Can you work these out from the model? Positions are in its coordinate system, mm. Face numbers are marked on the shaded views. A direction names the side the tool comes from. Give positions to 0.01 mm unless a question says otherwise; leave off trailing zeros. Order: outer loops, then holes, each group sorted by start corner. A loop starts at its lowest first (then second) coordinate and runs counter-clockwise, first axis right, second up.
Autodesk Inventor part; units mm, degrees
ref_plane "Work Plane1" through (0, 0, -15) normal (0, 0, 1) x (1, 0, 0)
ref_plane "YZ Plane" through (0, 0, 0) normal (1, 0, 0) x (0, 1, 0)
ref_plane "XZ Plane" through (0, 0, 0) normal (0, 1, 0) x (-1, 0, 0)
sketch "Sketch1" plane through (0, 0, 0) normal (0, 0, 1) x (1, 0, 0)
  line L0 (0, 0) -> (25, 0)
  line L1 (25, 0) -> (25, 40)
  line L2 (25, 40) -> (0, 40)
  line L3 (0, 40) -> (0, 0)
  dimension "d1" = 25
  dimension "d2" = 40
  dimension "d3" = 25
extrude "Extrusion1" add sketch "Sketch1" against normal blind 30
sketch "Sketch2" plane through (25, 0, 0) normal (1, 0, 0) x (0, 0, -1)
  line L0 (0, 0) -> (30, 0)
  circle A0 centre (15, 6.56) radius 2.46
extrude "Extrusion2" cut sketch "Sketch2" against normal blind 30
sketch "Sketch3" plane through (0, 0, 0) normal (-1, 0, 0) x (0, 0, 1)
  line L0 (0, 0) -> (-30, 0)
  line L1 (-25.05, 0) -> (-4.95, 0)
  line L2 (-4.95, 0) -> (-4.95, 33.12)
  line L3 (-4.95, 33.12) -> (-25.05, 33.12)
  line L4 (-25.05, 33.12) -> (-25.05, 0)
  dimension "d11" = 20.1
extrude "Extrusion3" cut sketch "Sketch3" against normal blind 20
sketch "Sketch4" plane through (0, 0, 0) normal (0, -1, 0) x (1, 0, 0)
  line L0 (20, -4.95) -> (20, -25.05)
  line L1 (20, -15) -> (25, -15)
  line L2 (25, 0) -> (25, -30)
  line L3 (20, -8.025) -> (25, -8.025)
  line L4 (25, -8.025) -> (25, -21.975)
  line L5 (25, -21.975) -> (20, -21.975)
  line L6 (20, -21.975) -> (20, -8.025)
  line L7 (20, -8.025) -> (25, -21.975) construction
  line L8 (25, -8.025) -> (20, -21.975) construction
  line L9 (25, -12.54) -> (25, -17.46)
  point P0 (0, 0)
  point P1 (22.5, -15)
  dimension "d14" = 13.95
extrude "Extrusion4" add sketch "Sketch4" along normal blind 15
sketch "Sketch5" plane through (20, 0, 0) normal (-1, 0, 0) x (0, 0, 1)
  circle A0 centre (-15, 6.56) radius 2.46
  circle A1 centre (-15, 6.56) radius 4.7025
  circle A2 centre (-15, 6.56) radius 2.46
  circle A3 centre (-15, 6.56) radius 2.46
  point P0 (0, 0)
  dimension "d17" = 9.405
extrude "Extrusion5" cut sketch "Sketch5" against normal blind 2.1
sketch "Sketch6" plane through (25, 0, 0) normal (1, 0, 0) x (0, 0, -1)
  circle A0 centre (15, 6.56) radius 4.7025
  line L0 (15, 6.56) -> (15, 23.56)
  circle A1 centre (15, 23.56) radius 2.46
  point P0 (0, 0)
  dimension "d20" = 17
  dimension "d21" = 4.92
extrude "Extrusion6" cut sketch "Sketch6" against normal blind 10 contours A1
sketch "Sketch7" plane through (20, 0, 0) normal (-1, 0, 0) x (0, 0, 1)
  circle A0 centre (-15, 23.56) radius 2.46
  circle A1 centre (-15, 23.56) radius 4.7025
  point P0 (0, 0)
  dimension "d24" = 9.405
extrude "Extrusion7" cut sketch "Sketch7" against normal blind 2.1
sketch "Sketch9" plane through (25, 0, 0) normal (1, 0, 0) x (0, 0, -1)
  circle A0 centre (15, 6.56) radius 2.46
  circle A1 centre (15, 6.56) radius 2.46
  circle A2 centre (15, 23.56) radius 2.46
  circle A3 centre (15, 23.56) radius 2.46
  line L0 (30, 40) -> (30, 0)
  line L1 (30, 0) -> (30, 40)
  line L2 (30, 40) -> (0, 40)
  line L3 (0, 40) -> (0, 0)
  line L4 (0, 0) -> (8.025, 0)
  line L5 (21.975, 0) -> (21.975, -15)
  line L6 (21.975, -15) -> (8.025, -15)
  line L7 (8.025, -15) -> (8.025, 0)
  line L8 (0, 0) -> (8.025, 0)
  line L9 (21.975, 0) -> (30, 0)
extrude "Extrusion8" add sketch "Sketch9" along normal blind 5
sketch "Sketch10" plane through (0, 40, 0) normal (0, 1, 0) x (1, 0, 0)
  line L0 (0, 30) -> (30, 30)
  line L1 (30, 0) -> (0, 0)
  line L2 (0, 30) -> (30, 30)
  line L3 (30, 30) -> (30, 0)
  line L4 (30, 0) -> (0, 0)
  line L5 (0, 0) -> (0, 30)
extrude "Extrusion9" add sketch "Sketch10" along normal blind 30
sketch "Sketch12" plane through (30, 0, 0) normal (1, 0, 0) x (0, 0, -1)
  circle A0 centre (15, 6.56) radius 2.46
  line L0 (15, 6.56) -> (15, 15.06)
  circle A1 centre (15, 15.06) radius 2.525
  point P0 (0, 0)
  dimension "d31" = 8.5
  dimension "d33" = 5.05
extrude "Extrusion10" cut sketch "Sketch12" against normal blind 30 contours A1
sketch "Sketch15" plane through (0, 0, -25.05) normal (-1, 0, 0) x (0, 0, 1)
  line L0 (0, 33.12) -> (20.1, 33.12)
  line L1 (20.1, 33.12) -> (20.1, 0)
  line L2 (0, 33.12) -> (20.1, 33.12)
  line L3 (20.1, 33.12) -> (20.1, 31.1)
  line L4 (20.1, 31.1) -> (0, 31.1)
  line L5 (0, 31.1) -> (0, 33.12)
  point P0 (25.05, 0)
  dimension "d57" = 2.02
extrude "Extrusion13" add sketch "Sketch15" against normal blind 20
sketch "Sketch17" plane through (0, 0, 0) normal (0, 0, 1) x (1, 0, 0)
  line L0 (0, 70) -> (30, 70)
  line L1 (30, 70) -> (50.0622, 90.0622)
  line L2 (30, 70) -> (80, 70) construction
  line L3 (11.9522, 97.2454) -> (0, 85.2932)
  line L4 (0, 70) -> (0, 85.2932)
  line L5 (0, 70) -> (0, 0)
  line L6 (0, 70) -> (30, 70)
  line L7 (10.923, 112.2849) -> (0, 120.567)
  line L8 (50.0622, 105.3553) -> (50.0622, 120.567)
  line L9 (50.0622, 105.3553) -> (50.0622, 90.0622)
  arc A0 (11.9522, 97.2454) -> (10.923, 112.2849) centre (4.8811, 104.3165) ccw
  line L10 (0, 165.567) -> (30, 165.567)
  line L11 (30, 165.567) -> (50.0622, 120.567)
  line L12 (6, 163.067) -> (0, 165.567)
  line L13 (6, 123.067) -> (0, 120.567)
  line L14 (6, 123.067) -> (12, 143.067)
  line L15 (12, 143.067) -> (6, 163.067)
  dimension "d61" = 45
  dimension "d62" = 32.0271
  dimension "d72" = 10
extrude "Extrusion14" add sketch "Sketch17" against normal blind 30
sketch "Sketch24" plane through (0, 0, 0) normal (0, 0, 1) x (1, 0, 0)
  line L0 (30, 70) -> (50.0622, 90.0622)
  line L1 (30, 70) -> (50.0622, 90.0622)
  line L2 (50.0622, 90.0622) -> (50.0622, 120.567)
  line L3 (50.0622, 90.0622) -> (50.0622, 120.567)
  line L4 (30, 165.567) -> (50.0622, 120.567)
  line L5 (50.0622, 120.567) -> (30, 165.567)
  line L6 (0, 165.567) -> (30, 165.567)
  line L7 (30, 165.567) -> (0, 165.567)
  line L8 (6, 163.067) -> (0, 165.567)
  line L9 (0, 165.567) -> (6, 163.067)
  line L10 (12, 143.067) -> (6, 163.067)
  line L11 (6, 163.067) -> (12, 143.067)
  line L12 (6, 123.067) -> (12, 143.067)
  line L13 (12, 143.067) -> (6, 123.067)
  line L14 (0, 120.567) -> (6, 123.067)
  line L15 (6, 123.067) -> (0, 120.567)
  line L16 (10.923, 112.2849) -> (0, 120.567)
  line L17 (0, 120.567) -> (10.923, 112.2849)
  line L18 (0, 85.2932) -> (11.9522, 97.2454)
  line L19 (11.9522, 97.2454) -> (0, 85.2932)
  line L20 (0, 85.2932) -> (0, 55.2932)
  line L21 (0, 0) -> (0, 85.2932)
  line L22 (0, 55.2932) -> (30, 55.2932)
  line L23 (30, 0) -> (30, 70)
  line L24 (30, 55.2932) -> (30, 70)
  arc A0 (11.9522, 97.2454) -> (10.923, 112.2849) centre (4.8811, 104.3165) ccw
  arc A1 (11.9522, 97.2454) -> (10.923, 112.2849) centre (4.8811, 104.3165) ccw
  dimension "d102" = 30
extrude "Extrusion15" add sketch "Sketch24" along normal blind 15
ref_plane "Work Plane1" through (0, 0, -15) normal (0, 0, 1) x (1, 0, 0)
mirror "Mirror1" about plane through (0, 0, -15) normal (0, 0, 1) of "Extrusion15"
properties part number "rec_c_40mm_x_60mm"
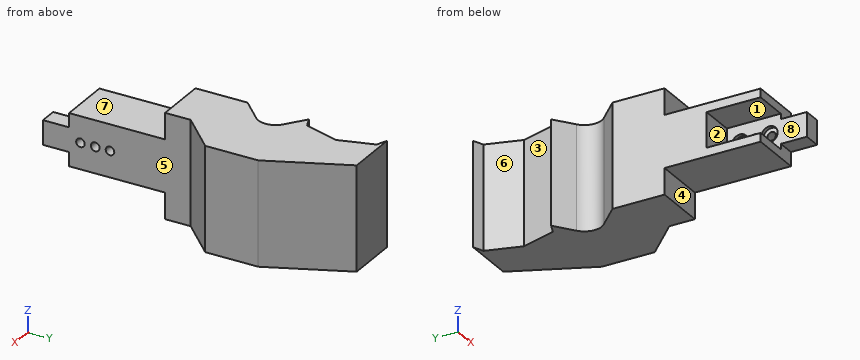
1) I'm going to push flat-ended pins straight in: pin 1 Ø9 at (x, y) = (14.5, 17) entering from -Z; pin 2 Ø4.5 at (x, z) = (22, -34.5) entering from -Y; pin 3 Ø5 at (x, y) = (23, -11) entering from -Z (3 decimals). Where does each tip first touch, or does it pass through?
2) We'd pull the mould along Y, two halves only. Please class the marked faces 1, 2 and 3: +Y half, -Y half, draft (parallel to the pull), parting line (faces both ways), or undercut.
3) Suppose I cut it at B-B (z = -38.5). Please give me the cut outline in (x, y), and give its area (3 significant figures).
4) Suppose I cut it at C-C (x = 17). Please give me the cut outline in (y, z), and give its area (3 significant figures).
5) Suppose I cut it at A-A (y = 23.56). Please give me the cut outline in (x, z).
6) If I drill on line 1 (Y direction, x = 28, z = -15) (3 decimals); line 2 (Y direction, x = 21, z = -15) (1 decimal); line 3 (Z direction, x = 21, y = 23), over which ranges is the centre line in solid material (lowest first)?
7) Suppose I cut it at D-D (z = -15). Give the number of separate pieces and of enclosed holes in the cut face, and give its area (3 significant figures).
8) Which directions (+Z, -Z, +X, -X, +Y, -Y) give clear straight access to the entire face, cutting with the end or side of a thin tool? Please do the marked faces 4, 5, 6, 7 and 8.
Results:
1. pin 1: stops at z = -30
1. pin 2: stops at y = 55.29
1. pin 3: stops at z = -21.975
2. face 1: draft
2. face 2: -Y half
2. face 3: undercut
3. outline: (0, 55.29) - (30, 55.29) - (30, 70) - (50.06, 90.06) - (50.06, 120.57) - (30, 165.57) - (0, 165.57) - (6, 163.07) - (12, 143.07) - (6, 123.07) - (0, 120.57) - (10.92, 112.28) arc R10 cw to (11.95, 97.25) - (0, 85.29) - close
3. area: 3,870 mm2
4. outline: (0, -30) - (55.29, -30) - (55.29, -45) - (165.57, -45) - (165.57, 15) - (55.29, 15) - (55.29, 0) - (0, 0) - (0, -4.95) - (31.1, -4.95) - (31.1, -25.05) - (0, -25.05) - close
4. area: 7,650 mm2
5. outline: (0, -30) - (30, -30) - (30, -17.46) - (22.1, -17.46) - (22.1, -19.7) - (20, -19.7) - (20, -25.05) - (0, -25.05) - close; (0, -4.95) - (20, -4.95) - (20, -10.3) - (22.1, -10.3) - (22.1, -12.54) - (30, -12.54) - (30, 0) - (0, 0) - close
6. line 1: y = -15 to 4.1, 9.02 to 12.535, 17.585 to 21.1, 26.02 to 165.567
6. line 2: y = -15 to 1.9, 11.3 to 12.5, 17.6 to 18.9, 28.3 to 165.6
6. line 3: z = -30 to -19.67, -10.33 to 0
7. separate pieces: 4
7. enclosed holes: 0
7. area: 4,890 mm2
8. face 4: -Z, +X, -X, -Y
8. face 5: +Z, -Z, +X, -Y
8. face 6: +Z, -Z, -X
8. face 7: +Z, +X, -X, -Y
8. face 8: -X, -Y
